CAD build for the part. Positions are in the model's coordinates, mm. A direction names the side the tool comes from. Coordinates: 2 decimals unless noted, no trailing zeros. Order: outer loops, then holes, each group sorted by start corner. A loop starts at its lowest first (then second) coordinate and runs counter-clockwise, first axis right, second up. Notation, with made-up numbers: (64, 8) - (78, 8) arc R11 cw to (78, 13) - close; hole circle Ø5 at (-13, 64). An arc over 180 degrees is marked (long way). Return JSON: item names as keys, results as strings.
from build123d import *

# Parameters (mm, degrees)
SKETCH1_W           = 25.4
SKETCH1_H           = 82.804
BOSS_EXTRUDE1_DEPTH = 33.274
SKETCH3_W           = 25.859634715
SKETCH3_H           = 25.4
BOSS_EXTRUDE2_DEPTH = 120.65
SKETCH4_W           = 25.4
SKETCH4_H           = 25.4
CUT_EXTRUDE2_DEPTH  = 25.4
SKETCH5_W           = 25.859634715
SKETCH5_H           = 9.652
BOSS_EXTRUDE3_DEPTH = 25.4
SKETCH7_R           = 3.175
CUT_EXTRUDE4_DEPTH  = 41.402
SKETCH8_R           = 3.175
CUT_EXTRUDE5_DEPTH  = 25.4
SKETCH6_R           = 3.175
CUT_EXTRUDE3_DEPTH  = 41.402
FILLET1_R           = 12.7
FILLET2_R           = 2.54


with BuildPart() as part:
    # Sketch1 → Boss-Extrude1 (new body)
    with BuildSketch(Plane(origin=(0, 0, 0), x_dir=(1, 0, 0), z_dir=(0, 1, 0))):
        with Locations((13.650196891, -15.542365285)):
            Rectangle(SKETCH1_W, SKETCH1_H)
    extrude(amount=BOSS_EXTRUDE1_DEPTH)

    # Sketch3 → Boss-Extrude2 (add)
    with BuildSketch(Plane(origin=(26.350196891, 0, 0), x_dir=(0, 0, -1), z_dir=(1, 0, 0))):
        with Locations((12.929817358, 20.574)):
            Rectangle(SKETCH3_W, SKETCH3_H)
    extrude(amount=BOSS_EXTRUDE2_DEPTH)

    # Sketch4 → Cut-Extrude2 (cut)
    with BuildSketch(Plane.XY.offset(56.944365285)):
        with Locations((13.650196891, 20.574)):
            Rectangle(SKETCH4_W, SKETCH4_H)
    extrude(amount=-CUT_EXTRUDE2_DEPTH, mode=Mode.SUBTRACT)

    # Sketch5 → Boss-Extrude3 (add)
    with BuildSketch(Plane(origin=(147.000196891, 0, 0), x_dir=(0, 0, -1), z_dir=(1, 0, 0))):
        with Locations((12.929817358, 20.574)):
            Rectangle(SKETCH5_W, SKETCH5_H)
    extrude(amount=BOSS_EXTRUDE3_DEPTH)

    # Sketch7 → Cut-Extrude4 (cut)
    with BuildSketch(Plane(origin=(0, 25.4, 0), x_dir=(1, 0, 0), z_dir=(0, 1, 0))):
        with Locations(Location((159.700196891, 12.929817358, 0), (0, 0, 270))):
            Circle(SKETCH7_R)
    extrude(amount=-CUT_EXTRUDE4_DEPTH, mode=Mode.SUBTRACT)

    # Sketch8 → Cut-Extrude5 (cut)
    with BuildSketch(Plane(origin=(0, 7.874, 0), x_dir=(1, 0, 0), z_dir=(0, 1, 0))):
        with Locations(Location((13.650196891, -44.244365285, 0), (0, 0, 270))):
            Circle(SKETCH8_R)
    extrude(amount=-CUT_EXTRUDE5_DEPTH, mode=Mode.SUBTRACT)

    # Sketch6 → Cut-Extrude3 (cut)
    with BuildSketch(Plane(origin=(0, 33.274, 0), x_dir=(1, 0, 0), z_dir=(0, 1, 0))):
        with Locations(Location((13.650196891, 12.929817358, 0), (0, 0, 270))):
            Circle(SKETCH6_R)
    extrude(amount=-CUT_EXTRUDE3_DEPTH, mode=Mode.SUBTRACT)

    # Fillet1
    fillet1_edges = [part.edges().sort_by_distance(p)[0] for p in [
        (0.950196891, 16.637, -25.859634715),
    ]]
    fillet(fillet1_edges, radius=FILLET1_R)

    # Fillet2
    fillet2_edges = [part.edges().sort_by_distance(p)[0] for p in [
        (26.350196891, 20.574, 0),
    ]]
    fillet(fillet2_edges, radius=FILLET2_R)


solid = part.part
Item 1: Band-saw the part on D-D, the plane x = 58.5. List the corners of the cut face in (y, z).
Findings below:
{"outline": "(7.87, -25.86) - (33.27, -25.86) - (33.27, 0) - (7.87, 0) - close"}
Item 2: Band-saw the part on A-A, the plane y = 11. List the corners of the cut face in (x, z) (3 decimals), then the cut area to 3 significant figures.
Findings below:
{"outline": "(0.95, -13.16) arc R12.7 ccw to (13.65, -25.86) - (147, -25.86) - (147, 0) - (28.89, 0) arc R2.54 cw to (26.35, 2.54) - (26.35, 31.544) - (0.95, 31.544) - close; hole circle Ø6.35 at (13.65, -12.93)", "area": "4,510 mm²"}
Item 3: Drop flat-ended pins along their axis: P1, Ø5, axis at y = 10, z = -2.5, coming from the +X side; P2, Ø12.5, axis at x = 75.5, y = 17, coming from the +Z side; P3, Ø5, axis at x = 13.65, z = -12.93, coming from the +Y side; P4, Ø12.5, axis at x = 166, z = -12.5, coming from the +Y side. Give the stop position or say it passes through.
Findings below:
{"P1": "stops at x = 147", "P2": "stops at z = 0", "P3": "passes through", "P4": "stops at y = 25.4"}
Item 4: Wall check: L1, parallel to X at y = 21, z = -13; L2, parallel to Z at x = 72.5, y = 14.5; L3, parallel to X at y = 18, z = 25.5. Give the ranges that are in metal, low to high. Write a range as [from, to].
Findings below:
{"L1": "x = [0.95, 10.48], [16.82, 156.53], [162.87, 172.4]", "L2": "z = [-25.86, 0]", "L3": "x = [0.95, 26.35]"}
Item 5: Which spindle directions (+Z, -Z, +X, -X, +Y, -Y) get a long thin tool onto all of the face, cutting with end or side? Do faces 1 (the flat face through (162, 25.4, -16)), 2 (the flat face through (86, 7.874, -11)), 3 (the flat face through (26.35, 13, 16)), 4 (the flat face through (16, 7.874, 47)), 5 (the flat face through (84, 20, 0)). Say none if no direction does.
Findings below:
{"face 1": "+Z, -Z, +X, +Y", "face 2": "+Z, -Z, +X, -Y", "face 3": "+Z, +X, -Y", "face 4": "+Z, +X, -X, +Y", "face 5": "+Z, +X, +Y, -Y"}
Item 6: Band-saw the part on C-C, the plane z = 13.5. List the corners of the cut face in (x, y), then the cut area to 3 significant figures.
Findings below:
{"outline": "(0.95, 0) - (26.35, 0) - (26.35, 33.27) - (0.95, 33.27) - close", "area": "845 mm²"}
Item 7: Band-saw the part on B-B, the plane y = 2. List the corners of the cut face in (x, z) (3 decimals).
Findings below:
{"outline": "(0.95, -13.16) arc R12.7 ccw to (13.65, -25.86) - (26.35, -25.86) - (26.35, 56.944) - (0.95, 56.944) - close; hole circle Ø6.35 at (13.65, -12.93); hole circle Ø6.35 at (13.65, 44.244)"}
